from build123d import *

# Parameters (mm, degrees)
SKETCH1_W           = 116
SKETCH1_H           = 54
SKETCH1_R           = 2.05
SKETCH1_R_2         = 7
BOSS_EXTRUDE1_DEPTH = 3.175
FILLET1_R           = 4


with BuildPart() as part:
    # Sketch1 → Boss-Extrude1 (new body)
    with BuildSketch(Plane.XY):
        Rectangle(SKETCH1_W, SKETCH1_H)
        with Locations((-53.195, 22)):
            Circle(SKETCH1_R, mode=Mode.SUBTRACT)
        with Locations((53.195, 22)):
            Circle(SKETCH1_R, mode=Mode.SUBTRACT)
        with Locations((53.195, -22)):
            Circle(SKETCH1_R, mode=Mode.SUBTRACT)
        with Locations((-53.195, -22)):
            Circle(SKETCH1_R, mode=Mode.SUBTRACT)
        with Locations((-39.195, 8)):
            Circle(SKETCH1_R, mode=Mode.SUBTRACT)
        with Locations((-23.195, 8)):
            Circle(SKETCH1_R, mode=Mode.SUBTRACT)
        with Locations((-23.195, -8)):
            Circle(SKETCH1_R, mode=Mode.SUBTRACT)
        with Locations((-39.195, -8)):
            Circle(SKETCH1_R, mode=Mode.SUBTRACT)
        with Locations((-31.195, 0)):
            Circle(SKETCH1_R_2, mode=Mode.SUBTRACT)
        with Locations(Location((39.195, -8, 0), (0, 0, 180))):
            Circle(SKETCH1_R, mode=Mode.SUBTRACT)
        with Locations(Location((39.195, 8, 0), (0, 0, 180))):
            Circle(SKETCH1_R, mode=Mode.SUBTRACT)
        with Locations(Location((23.195, 8, 0), (0, 0, 180))):
            Circle(SKETCH1_R, mode=Mode.SUBTRACT)
        with Locations(Location((31.195, 0, 0), (0, 0, 180))):
            Circle(SKETCH1_R_2, mode=Mode.SUBTRACT)
        with Locations(Location((23.195, -8, 0), (0, 0, 180))):
            Circle(SKETCH1_R, mode=Mode.SUBTRACT)
    extrude(amount=BOSS_EXTRUDE1_DEPTH)

    # Fillet1
    fillet1_edges = [part.edges().sort_by_distance(p)[0] for p in [
        (-58, 27, 1.5875),
        (58, 27, 1.5875),
        (58, -27, 1.5875),
        (-58, -27, 1.5875),
    ]]
    fillet(fillet1_edges, radius=FILLET1_R)


solid = part.part
Design review of the part built by this model. Coordinates are the model's own, in mm. Coordinates: 2 decimals unless noted, no trailing zeros. Order: outer loops, then holes, each group sorted by start corner. A loop starts at its lowest first (then second) coordinate and runs counter-clockwise, first axis right, second up. Notation, with made-up numbers: (2, 11) -> (51, 11) arc R23 cw to (51, 20) -> close; hole circle Ø3 at (-32.75, 16). An arc over 180 degrees is marked (long way). Use one line per item in the form item = value. Start each with the question number.
(1) For probe 1 along Y at (x, z) = (-52, 1.8); probe 2 along Y at (x, z) = (-21.5, 2.8); probe 3 along Y at (x, z) = (-25, 2.1), list the stretches that pass through material, from the lowest coordinate up.
(2) The part is to be moulded in two halves that separate along X. For faces 1 (the flat face through (58, 0, 2)), 2 (the cylindrical face through (41.243, 7.91, 1.565)), 3 (the flat face through (-1, 27, 2)), say which applies: +X half, -X half, draft (parallel to the pull), parting line (faces both ways), or undercut.
(3) Add section C-C on y = -4.5. State the section outline as (x, z) points (3 decimals).
(4) Add section A-A on z = 1.15. Give the number of separate pieces and of enclosed holes in the cut face, plus the area to 3 significant figures.
(5) Add section B-B on x = 31. State the section outline as (y, z) points (3 decimals).
Answer block:
q1.probe_1 = -27 to -23.67, -20.33 to 20.33, 23.67 to 27
q1.probe_2 = -27 to -9.15, -6.85 to 6.85, 9.15 to 27
q1.probe_3 = -27 to -8.97, -7.03 to -3.26, 3.26 to 7.03, 8.97 to 27
q2.face_1 = +X half
q2.face_2 = undercut
q2.face_3 = draft
q3.outline = (-58, 0) -> (-36.557, 0) -> (-36.557, 3.175) -> (-58, 3.175) -> close; (-25.833, 0) -> (25.833, 0) -> (25.833, 3.175) -> (-25.833, 3.175) -> close; (36.557, 0) -> (58, 0) -> (58, 3.175) -> (36.557, 3.175) -> close
q4.separate_pieces = 1
q4.enclosed_holes = 14
q4.area = 5,780 mm²
q5.outline = (-27, 0) -> (-6.997, 0) -> (-6.997, 3.175) -> (-27, 3.175) -> close; (6.997, 0) -> (27, 0) -> (27, 3.175) -> (6.997, 3.175) -> close
